```python
from build123d import *

# Parameters (mm, degrees)
SKETCH1_W           = 30
SKETCH1_H           = 30
BOSS_EXTRUDE1_DEPTH = 12
SKETCH2_W           = 5
SKETCH2_H           = 12
SKETCH2_W_2         = 8
BOSS_EXTRUDE2_DEPTH = 25
FILLET1_R           = 8
SKETCH3_R           = 2.15
CUT_EXTRUDE1_DEPTH  = 50.939963957


with BuildPart() as part:
    # Sketch1 → Boss-Extrude1 (new body)
    with BuildSketch(Plane(origin=(0, 0, 0), x_dir=(1, 0, 0), z_dir=(0, 1, 0))):
        Rectangle(SKETCH1_W, SKETCH1_H)
    extrude(amount=BOSS_EXTRUDE1_DEPTH)

    # Sketch2 → Boss-Extrude2 (add)
    with BuildSketch(Plane(origin=(0, 12, 0), x_dir=(1, 0, 0), z_dir=(0, 1, 0))):
        with Locations((12.5, 0)):
            Rectangle(SKETCH2_W, SKETCH2_H)
        with Locations((6, 0)):
            Rectangle(SKETCH2_W_2, SKETCH2_H)
    extrude(amount=BOSS_EXTRUDE2_DEPTH)

    # Fillet1
    fillet1_edges = [part.edges().sort_by_distance(p)[0] for p in [
        (8.5, 12, -6),
        (8.5, 12, 6),
    ]]
    fillet(fillet1_edges, radius=FILLET1_R)

    # Sketch3 → Cut-Extrude1 (cut, through all)
    with BuildSketch(Plane(origin=(15, 0, 0), x_dir=(0, 0, -1), z_dir=(1, 0, 0))):
        with Locations((0, 17)):
            Circle(SKETCH3_R)
        with Locations((0, 32)):
            Circle(SKETCH3_R)
    extrude(amount=-CUT_EXTRUDE1_DEPTH, mode=Mode.SUBTRACT)


solid = part.part
```
Here's how the part is built. I have some questions about the finished solid (model axes, mm). A direction names the side the tool comes from. Give positions to 0.01 mm unless a question says otherwise; leave off trailing zeros. Loops run counter-clockwise (first coordinate to the right, second up) from the corner with the lowest first, then second, coordinate; pieces in that order, holes last. Notation, with made-up numbers: M 10,-5.75 L 53,-5.75 A17 cw 53,3.25 Z; hole C 61.25,-4 d1. An arc over 180 degrees is marked long. Put each result on its own line as item: value. Start each with the question number.
(1) If we mould it in two halves opening along Y, with no side actions, what happens to faces 1 (the flat face through (-7, 12, 0)), 2 (the cylindrical face through (8.59, 14.9, 0.47)), 3 (the flat face through (2, 22, 0))? For each: +Y half, -Y half, draft (parallel to the pull), parting line (faces both ways), or undercut.
(2) I want a section at D-D on z = -3.5. Please give me the cut outline in (x, y).
(3) I want a section at B-B on y = 17. Please give me the cut outline in (x, z), then the cut area to 3 significant figures.
(4) I need wall thicknesses on line 1 along Y through (x, z) = (11.25, 0); line 2 along X through (y, z) = (15, -1); line 3 along Y through (x, z) = (-4.25, -9.5). Which ranges of each line are inside material? Lowest first, please. Write a range as [from, to].
(5) I want a section at C-C on x = 9.5. Please give me the cut outline in (y, z).
(6) For faces 4 (the flat face through (9, 28, -6)), 5 (the flat face through (0, 0, 0)), 6 (the flat face through (8, 28, 6)), which set-ups out of +Z, -Z, +X, -X, +Y, -Y let a thin tool reach every point of the face, with its end or its side?
(7) Will these pins go through, and if not, where does the flat tip stop? pin 1 Ø4 at (y, z) = (17, 0) entering from -X; pin 2 Ø14.5 at (x, y) = (11, 30.5) entering from -Z; pin 3 Ø1 at (y, z) = (30, 4.5) entering from -X; pin 4 Ø4 at (x, y) = (5.5, 27) entering from +Z.
(8) I want a section at A-A on z = 0. Please give me the cut outline in (x, y), then the cut area to 3 significant figures.
Answer block:
1. face 1: +Y half
1. face 2: undercut
1. face 3: draft
2. outline: M -15,0 L 15,0 L 15,37 L 2,37 L 2,12 L -15,12 Z
3. outline: M 2,-6.58 L 15,-6.58 L 15,-2.15 L 2,-2.15 Z; M 2,2.15 L 15,2.15 L 15,6.58 L 2,6.58 Z
3. area: 115 mm^2
4. line 1: [0, 14.85], [19.15, 29.85], [34.15, 37]
4. line 2: [2, 15]
4. line 3: [0, 12]
5. outline: M 0,-15 L 12,-15 L 12,-14 A8 cw 20,-6 L 37,-6 L 37,6 L 20,6 A8 cw 12,14 L 12,15 L 0,15 Z; hole C 17,0 d4.3; hole C 32,0 d4.3
6. face 4: -Z, +X, -X, +Y
6. face 5: +Z, -Z, +X, -X, -Y
6. face 6: +Z, +X, -X, +Y
7. pin 1: through
7. pin 2: z = -6
7. pin 3: x = 2
7. pin 4: z = 6
8. outline: M -15,0 L 15,0 L 15,14.85 L 2,14.85 L 2,12 L -15,12 Z; M 2,19.15 L 15,19.15 L 15,29.85 L 2,29.85 Z; M 2,34.15 L 15,34.15 L 15,37 L 2,37 Z
8. area: 573 mm^2
